Could you check a few things on this model? Use its own coordinates, in mm. A direction names the side the tool comes from. Round coordinates to 2 decimals unless told otherwise and drop trailing zeros. Loops run counter-clockwise (first coordinate to the right, second up) from the corner with the lowest first, then second, coordinate; pieces in that order, holes last. Notation, with made-up numbers: (56.5, 9) - (67.5, 9) arc R34 cw to (67.5, 42) - close; hole circle Ø2 at (-7.5, 76.5). An arc over 180 degrees is marked (long way). Answer as CSV lines item,"result". Start each with the question number.
1) We'd pull the mould along Y, two halves only. Please class faces 1 (the face through (25, 51, 0)), 2 (the face through (24.45, 124.994, 4.958)), 3 (the face through (20, 0, 4)): pulls with the +Y half, pulls with the -Y half, needs draft (parallel to the pull), parting line crosses it, or undercut.
2) Suppose I cut it at A-A, the plane y = 97. Write out the boundary of the cut face in (x, z), then the cut area to 3 significant figures.
3) Please list where these lines run through material, in increasing order: line 1 along Y through (x, z) = (36, 6); line 2 along X through (y, z) = (-11.5, 3.75); line 3 along X through (y, z) = (87.5, 6.5).
4) Suppose I cut it at B-B, the plane y = -6.5. Count the separate pieces of the cut face and the enclosed holes in it, then the cut area to 3 significant figures.
5) I'm going to push flat-ended pins straight in: pin 1 Ø7 at (x, y) = (29.45, -12.22) entering from +Z; pin 2 Ø5 at (x, z) = (31.5, 5.5) entering from +Y; pin 3 Ø3 at (x, z) = (29.5, 3) entering from +Y. Where does each tip first touch, or does it pass through?
6) Which directions (+Z, -Z, +X, -X, +Y, -Y) give clear straight access to the entire face, cutting with the end or side of a thin tool? Please do faces 4 (the face through (23.7, 11.7, 2)), 5 (the face through (25.55, -24.994, 4.958)), 6 (the face through (26.46, 88.39, 5.07)).
```python
from build123d import *

# Parameters (mm, degrees)
SKETCH1_R           = 5
BOSS_EXTRUDE1_DEPTH = 10
CUT_EXTRUDE2_DEPTH  = 10
FILLET1_R           = 2
FILLET2_R           = 2
SKETCH3_R           = 18.1
CUT_EXTRUDE3_DEPTH  = 2
SKETCH4_R           = 1.5
CUT_EXTRUDE4_DEPTH  = 136.000000037
SKETCH4_3_R         = 3
SKETCH4_3_R_2       = 1.5
CUT_EXTRUDE5_DEPTH  = 2
CIRPATTERN1_COUNT   = 9


with BuildPart() as part:
    # Sketch1 → Boss-Extrude1 (new body)
    # profile 1 of 2: a face of its own
    with BuildSketch(Plane.XY):
        with BuildLine():
            Line((0, 0), (0, 100))
            ThreePointArc((0, 100), (25, 125), (50, 100))
            Line((50, 100), (50, 0))
            ThreePointArc((50, 0), (25, -25), (0, 0))
        make_face()
        with BuildLine():
            ThreePointArc((15, 0), (25, -10), (35, 0))
            Line((35, 0), (35, 100))
            ThreePointArc((35, 100), (25, 110), (15, 100))
            Line((15, 100), (15, 0))
        make_face(mode=Mode.SUBTRACT)
    # profile 2 of 2: a face of its own
    with BuildSketch(Plane.XY):
        with BuildLine():
            Line((15, 0), (15, 100))
            ThreePointArc((15, 100), (25, 110), (35, 100))
            Line((35, 100), (35, 0))
            ThreePointArc((35, 0), (25, -10), (15, 0))
        make_face()
        with Locations((25, 0)):
            Circle(SKETCH1_R, mode=Mode.SUBTRACT)
        with Locations((25, 100)):
            Circle(SKETCH1_R, mode=Mode.SUBTRACT)
    extrude(amount=BOSS_EXTRUDE1_DEPTH)

    # Sketch2 → Cut-Extrude2 (cut)
    with BuildSketch(Plane.XY.offset(10)):
        with BuildLine():
            Line((25.064971157, 89.343145751), (10, 89.343145751))
            Line((10, 89.343145751), (10, 70.656854249))
            Line((10, 70.656854249), (26.125631329, 86.782485579))
            ThreePointArc((26.125631329, 86.782485579), (26.450790456, 88.417170899), (25.064971157, 89.343145751))
        make_face()
        with BuildLine():
            Line((40, 69), (40, 89.343145751))
            Line((40, 89.343145751), (22.217514421, 71.560660172))
            ThreePointArc((22.217514421, 71.560660172), (21.892355294, 69.925974851), (23.278174593, 69))
            Line((23.278174593, 69), (40, 69))
        make_face()
        with BuildLine():
            Line((26.721825407, 61), (10, 61))
            Line((10, 61), (10, 40.65685425))
            Line((10, 40.65685425), (22.171572875, 52.828427125))
            Line((22.171572875, 52.828427125), (27.782485579, 58.439339828))
            ThreePointArc((27.782485579, 58.439339828), (28.107644706, 60.074025149), (26.721825407, 61))
        make_face()
        with BuildLine():
            Line((40, 39), (40, 59.343145751))
            Line((40, 59.343145751), (27.828427125, 47.171572875))
            Line((27.828427125, 47.171572875), (22.217514421, 41.560660172))
            ThreePointArc((22.217514421, 41.560660172), (21.892355294, 39.925974852), (23.278174593, 39))
            Line((23.278174593, 39), (40, 39))
        make_face()
    extrude(amount=-CUT_EXTRUDE2_DEPTH, mode=Mode.SUBTRACT)

    # Fillet1
    fillet1_edges = [part.edges().sort_by_distance(p)[0] for p in [
        (40, 89.343145751, 5),
        (40, 69, 5),
        (10, 40.65685425, 5),
        (10, 61, 5),
        (40, 59.343145751, 5),
        (40, 39, 5),
        (10, 70.656854249, 5),
        (10, 89.343145751, 5),
    ]]
    fillet(fillet1_edges, radius=FILLET1_R)

    # Fillet2
    fillet2_edges = [part.edges().sort_by_distance(p)[0] for p in [
        (25, -25, 0),
        (0, 50, 0),
        (25, -25, 10),
        (50, 50, 10),
        (25, 125, 10),
        (0, 50, 10),
        (25, 125, 0),
        (50, 50, 0),
    ]]
    fillet(fillet2_edges, radius=FILLET2_R)

    # Sketch3 → Cut-Extrude3 (cut)
    with BuildSketch(Plane.XY.offset(10)):
        with Locations((25, 0)):
            Circle(SKETCH3_R)
    extrude(amount=-CUT_EXTRUDE3_DEPTH, mode=Mode.SUBTRACT)

    # Sketch4 → Cut-Extrude4 (cut, through all)
    with BuildSketch(Plane(origin=(0, 0, 0), x_dir=(-1, 0, 0), z_dir=(0, 0, -1))):
        with Locations((-25, 13)):
            Circle(SKETCH4_R)
    cut_extrude4 = extrude(amount=-CUT_EXTRUDE4_DEPTH, mode=Mode.SUBTRACT)

    # Sketch4_3 → Cut-Extrude5 (cut)
    with BuildSketch(Plane(origin=(0, 0, 0), x_dir=(-1, 0, 0), z_dir=(0, 0, -1))):
        with Locations((-25, 13)):
            Circle(SKETCH4_3_R)
        with Locations((-25, 13)):
            Circle(SKETCH4_3_R_2, mode=Mode.SUBTRACT)
    cut_extrude5 = extrude(amount=-CUT_EXTRUDE5_DEPTH, mode=Mode.SUBTRACT)

    # CirPattern1: Cut-Extrude4, Cut-Extrude5 ×9 about axis
    cirpattern1_axis = Axis((25, 0, 0), (0, 0, 1))
    add([cut_extrude4.rotate(cirpattern1_axis, i * 360 / CIRPATTERN1_COUNT) for i in range(1, CIRPATTERN1_COUNT)], mode=Mode.SUBTRACT)
    add([cut_extrude5.rotate(cirpattern1_axis, i * 360 / CIRPATTERN1_COUNT) for i in range(1, CIRPATTERN1_COUNT)], mode=Mode.SUBTRACT)


solid = part.part
```
Filled sheet:
1,face 1,"needs draft"
1,face 2,"pulls with the +Y half"
1,face 3,"undercut"
2,outline,"(0, 2) arc R2 ccw to (2, 0) - (21, 0) - (21, 10) - (2, 10) arc R2 ccw to (0, 8) - close; (29, 0) - (48, 0) arc R2 ccw to (50, 2) - (50, 8) arc R2 ccw to (48, 10) - (29, 10) - close"
2,area,"417 mm²"
3,line 1,"-22.45 to -7.98, -5.02 to 39, 55.34 to 69, 85.34 to 122.45"
3,line 2,"2.8 to 19.24, 21.87 to 28.13, 30.76 to 47.2"
3,line 3,"0 to 10.01, 26.53 to 50"
4,separate pieces,"3"
4,enclosed holes,"0"
4,area,"352 mm²"
5,pin 1,"z = 8"
5,pin 2,"y = 124.68"
5,pin 3,"y = 124.82"
6,face 4,"-Z"
6,face 5,"+Z, -Z, -Y"
6,face 6,"+Z, -Z"
